```python
from build123d import *

# Parameters (mm, degrees)
F0_W     = 123
F0_H     = 36
F0_R     = 11
F1_DEPTH = 5
F2_DEPTH = 14
F3_SIZE  = 3
F4_ANGLE = 180


with BuildPart() as f1:
    # F0 (on Top) → F1 (new body)
    with BuildSketch(Plane.XY):
        with Locations((-0.073285, 7.507721)):
            Rectangle(F0_W, F0_H)
        with Locations((-43.573285, 7.507721)):
            Circle(F0_R, mode=Mode.SUBTRACT)
        with Locations((-14.573285, 7.507721)):
            Circle(F0_R, mode=Mode.SUBTRACT)
        with Locations((14.426715, 7.507721)):
            Circle(F0_R, mode=Mode.SUBTRACT)
        with Locations((43.426715, 7.507721)):
            Circle(F0_R, mode=Mode.SUBTRACT)
        with Locations((-43.573285, 7.507721)):
            Circle(F0_R)
        with Locations((-14.573285, 7.507721)):
            Circle(F0_R)
        with Locations((14.426715, 7.507721)):
            Circle(F0_R)
        with Locations((43.426715, 7.507721)):
            Circle(F0_R)
    extrude(amount=F1_DEPTH)

    # F0 (on Top) → F2 (join)
    with BuildSketch(Plane.XY):
        with Locations((-43.573285, 7.507721)):
            Circle(F0_R)
        with Locations((-14.573285, 7.507721)):
            Circle(F0_R)
        with Locations((14.426715, 7.507721)):
            Circle(F0_R)
        with Locations((43.426715, 7.507721)):
            Circle(F0_R)
    extrude(amount=-F2_DEPTH)

    # F3
    f3_edges = [f1.edges().sort_by_distance(p)[0] for p in [
        (-0.073285, 25.507721, 0),
        (-61.573285, 7.507721, 0),
        (61.426715, 7.507721, 0),
        (-0.073285, -10.492279, 0),
        (32.426715, 7.507721, -14),
        (3.426715, 7.507721, -14),
        (-25.573285, 7.507721, -14),
        (-54.573285, 7.507721, -14),
    ]]
    chamfer(f3_edges, length=F3_SIZE)


with BuildPart() as f1_1:
    # F4: moved
    add(f1.part.rotate(Axis((-0.073285, 7.507721, 0), (1, 0, 0)), F4_ANGLE))


solid = f1_1.part
```
Verification items for the finished model (mm, model axes). A direction names the side the tool comes from. Coordinates: 2 decimals unless noted, no trailing zeros. Write each loop counter-clockwise with the first axis right and the second up, starting at its lowest first coordinate (ties: lowest second). Pieces come first, ordered by that corner, then holes. Notation, with made-up numbers: (-3, 3) - (13, 3) arc R19 ccw to (13, 40) - close; hole circle Ø7 at (-27.75, -36). An arc over 180 degrees is marked (long way). One line per question, with ' | ' between items. Start each with the question number.
1. Draft check along X on faces 3 (the flat face through (59.948, 7.76, -1.521)), 4 (the flat face through (14, 7, 14)), 5 (the cylindrical face through (32.437, 7.024, 5.423)), 6 (the conical face through (-6.8, 5.06, 13.85)). Enter one of: released by +X, released by -X, zero draft, split by the parting line, or undercut.
2. Section check B-B (z = -1.5). Enter the section's corners in (x, y), plus the area to 3 significant figures.
3. Gauge pin test, flat ends, axial feed: P1, Ø9, axis at x = -4.5, y = 13, coming from the +Z side; P2, Ø1, axis at y = -3, z = 5.5, coming from the +X side; P3, Ø1, axis at x = -35.5, z = 4, coming from the +Y side; P4, Ø3, axis at y = 13, z = 6.5, coming from the +X side. Record the tip position at first contact, or that the pin passes through.
4. Section check A-A (z = 9). Enter the section's corners in (x, y).
5. Material ranges on line 1 along X through (y, z) = (8, 6); line 2 along Z through (x, y) = (52, -5.5); line 3 along X through (y, z) = (13, 10), recorded low to high.
6. Access from +Z, -Z, +X, -X, +Y, -Y to the whole of each face (thin tool, end or side, straight path). Record for faces 1 (the flat face through (43, 7, 14)), 2 (the cylindrical face through (24.919, 4.204, 5.423)).
Computed values:
1) face 3: released by +X | face 4: zero draft | face 5: undercut | face 6: undercut
2) outline: (-60.07, -8.99) - (59.93, -8.99) - (59.93, 24.01) - (-60.07, 24.01) - close | area: 3,960 mm²
3) P1: z = 14 | P2: x = 47.99 | P3: y = 15.49 | P4: x = 53.68
4) outline: circle Ø22 at (-43.57, 7.51); circle Ø22 at (-14.57, 7.51); circle Ø22 at (14.43, 7.51); circle Ø22 at (43.43, 7.51)
5) line 1: -54.56 to -32.58, -25.56 to -3.58, 3.44 to 25.42, 32.44 to 54.42 | line 2: -5 to 0 | line 3: -53.1 to -34.04, -24.1 to -5.04, 4.9 to 23.96, 33.9 to 52.96
6) face 1: +Z, +X, -X, +Y, -Y | face 2: +Z
